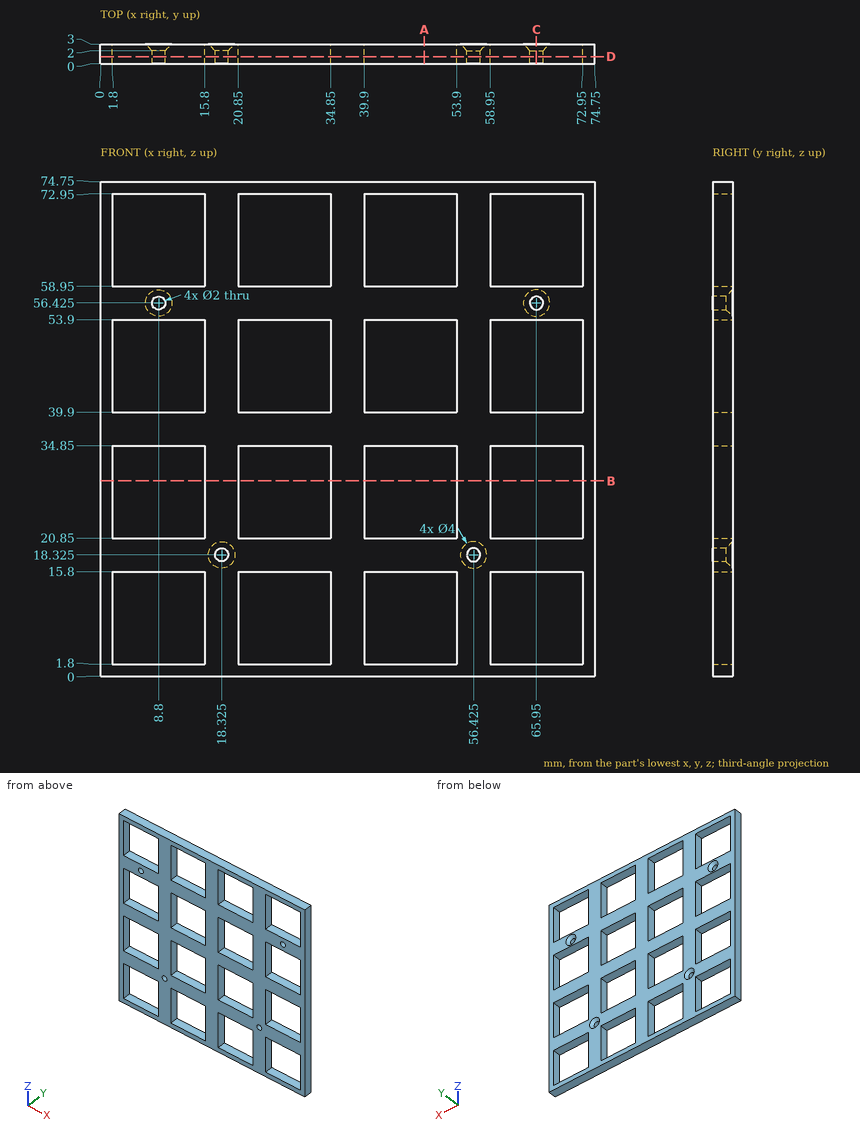
Can you work these out from the drawing? Everything is in mm from the part's minimum corner. Round coordinates to 2 decimals unless told otherwise and drop trailing zeros. Loops run counter-clockwise (first coordinate to the right, second up) from the corner with the lowest first, then second, coordinate; pieces in that order, holes last. Notation, with made-up numbers: (82.25, 43) -> (128.25, 43) arc R21 cw to (128.25, 60) -> close; hole circle Ø2 at (-24, 40.5). An arc over 180 degrees is marked (long way). Put each result on its own line as item: value.
Q1. I want a section at B-B on z = 29.5. Write out the boundary of the cut face in (x, y), and give its area (4 significant figures).
Checks:
outline: (0, 0) -> (1.8, 0) -> (1.8, 3) -> (0, 3) -> close; (15.8, 0) -> (20.85, 0) -> (20.85, 3) -> (15.8, 3) -> close; (34.85, 0) -> (39.9, 0) -> (39.9, 3) -> (34.85, 3) -> close; (53.9, 0) -> (58.95, 0) -> (58.95, 3) -> (53.9, 3) -> close; (72.95, 0) -> (74.75, 0) -> (74.75, 3) -> (72.95, 3) -> close
area: 56.25 mm2
Q2. For pin 1 Ø1.5 at (x, y) = (68, 1) entering from -Z, with a flat end and sliding along its axis, tell me the tip position at first contact or that it passes through.
Checks:
pin 1: z = 0
Q3. I want a section at D-D on y = 1.1. Give the number of separate pieces and of enclosed holes in the cut face, and give its area (3 significant figures).
Checks:
separate pieces: 1
enclosed holes: 20
area: 2,440 mm2
Q4. I want a section at C-C on x = 65.95. Write out the boundary of the cut face in (y, z) (3 decimals).
Checks:
outline: (0, 0) -> (3, 0) -> (3, 1.8) -> (0, 1.8) -> close; (0, 15.8) -> (3, 15.8) -> (3, 20.85) -> (0, 20.85) -> close; (0, 34.85) -> (3, 34.85) -> (3, 39.9) -> (0, 39.9) -> close; (0, 53.9) -> (3, 53.9) -> (3, 54.425) -> (2, 55.425) -> (0, 55.425) -> close; (0, 57.425) -> (2, 57.425) -> (3, 58.425) -> (3, 58.95) -> (0, 58.95) -> close; (0, 72.95) -> (3, 72.95) -> (3, 74.75) -> (0, 74.75) -> close
Q5. Please list where these lines run through material, in increasing order: line 1 (X direction, y = 0.8, z = 27); line 2 (Z direction, x = 65.95, y = 1.55) (3 decimals). Write a range as from..to.
Checks:
line 1: 0..1.8, 15.8..20.85, 34.85..39.9, 53.9..58.95, 72.95..74.75
line 2: 0..1.8, 15.8..20.85, 34.85..39.9, 53.9..55.425, 57.425..58.95, 72.95..74.75
Q6. I want a section at A-A on x = 49. Write out the boundary of the cut face in (y, z).
Checks:
outline: (0, 0) -> (3, 0) -> (3, 1.8) -> (0, 1.8) -> close; (0, 15.8) -> (3, 15.8) -> (3, 20.85) -> (0, 20.85) -> close; (0, 34.85) -> (3, 34.85) -> (3, 39.9) -> (0, 39.9) -> close; (0, 53.9) -> (3, 53.9) -> (3, 58.95) -> (0, 58.95) -> close; (0, 72.95) -> (3, 72.95) -> (3, 74.75) -> (0, 74.75) -> close
